```python
from build123d import *

# Parameters (mm, degrees)
SKETCH1_W           = 22.5
SKETCH1_H           = 17.75
SKETCH1_W_2         = 52
SKETCH1_H_2         = 71.85
BOSS_EXTRUDE1_DEPTH = 2
BOSS_EXTRUDE2_DEPTH = 3
SKETCH1_4_W         = 80.4
SKETCH1_4_H         = 94.4
SKETCH1_4_W_2       = 76
SKETCH1_4_H_2       = 90
BOSS_EXTRUDE3_DEPTH = 26
BOSS_EXTRUDE4_DEPTH = 78.2
CUT_EXTRUDE1_START  = -78.2
SKETCH2_3_W         = 10.3
SKETCH2_3_H         = 9
CUT_EXTRUDE1_DEPTH  = 26
CUT_EXTRUDE2_DEPTH  = 26
FILLET1_R           = 1.5
SKETCH4_R           = 3
CUT_EXTRUDE3_DEPTH  = 26
SKETCH5_R           = 1.6
BOSS_EXTRUDE5_DEPTH = 6
FILLET2_R           = 1.5


with BuildPart() as part:
    # Sketch1 → Boss-Extrude1 (new body)
    with BuildSketch(Plane(origin=(0, 0, 0), x_dir=(1, 0, 0), z_dir=(0, 1, 0))):
        Polygon((-38, -26.85), (-14, -26.85), (-14, 45), (-15.5, 45), (-15.5, 27.25), (-38, 27.25), align=None)
        with Locations((-26.75, 36.125)):
            Rectangle(SKETCH1_W, SKETCH1_H)
        with Locations((12, 9.075)):
            Rectangle(SKETCH1_W_2, SKETCH1_H_2)
        Polygon((38, -45), (38, -26.85), (-14, -26.85), (-38, -26.85), (-38, -45), align=None)
    extrude(amount=BOSS_EXTRUDE1_DEPTH)

    # Sketch1<3> → Boss-Extrude2 (add)
    with BuildSketch(Plane(origin=(0, 0, 0), x_dir=(1, 0, 0), z_dir=(0, 1, 0))):
        Polygon((-38, -26.85), (-14, -26.85), (-14, 45), (-15.5, 45), (-15.5, 27.25), (-38, 27.25), align=None)
    extrude(amount=BOSS_EXTRUDE2_DEPTH)

    # Sketch1<4> → Boss-Extrude3 (add)
    with BuildSketch(Plane(origin=(0, 0, 0), x_dir=(1, 0, 0), z_dir=(0, 1, 0))):
        Rectangle(SKETCH1_4_W, SKETCH1_4_H)
        Rectangle(SKETCH1_4_W_2, SKETCH1_4_H_2, mode=Mode.SUBTRACT)
    extrude(amount=BOSS_EXTRUDE3_DEPTH)

    # Sketch2 → Boss-Extrude4 (add)
    with BuildSketch(Plane.ZY.offset(40.2)):
        with BuildLine():
            Line((28.764343606, 5.5), (26.964343606, 5.5))
            Line((26.964343606, 5.5), (26.964343606, 0))
            Line((26.964343606, 0), (41.904953918, 0))
            Line((41.904953918, 0), (47.2, 0))
            Line((47.2, 0), (47.2, 5.5375))
            Line((47.2, 5.5375), (45, 5.5375))
            Line((45, 5.5375), (43.114695317, 5.5375))
            ThreePointArc((43.114695317, 5.5375), (35.948714495, 2.000030985), (28.764343606, 5.5))
        make_face()
    extrude(amount=-BOSS_EXTRUDE4_DEPTH)

    # Sketch2<3> → Cut-Extrude1 (cut)
    with BuildSketch(Plane.ZY.offset(40.2).offset(CUT_EXTRUDE1_START)):
        with Locations((10.914343606, 17.8)):
            Rectangle(SKETCH2_3_W, SKETCH2_3_H)
    extrude(amount=-CUT_EXTRUDE1_DEPTH, mode=Mode.SUBTRACT)

    # Sketch3 → Cut-Extrude2 (cut)
    with BuildSketch(Plane.ZY.offset(40.2)):
        with BuildLine():
            Line((-39.125, 8.5), (-33.125, 8.5))
            ThreePointArc((-33.125, 8.5), (-30.375, 5.75), (-33.125, 3))
            Line((-33.125, 3), (-39.125, 3))
            ThreePointArc((-39.125, 3), (-41.875, 5.75), (-39.125, 8.5))
        make_face()
    extrude(amount=-CUT_EXTRUDE2_DEPTH, mode=Mode.SUBTRACT)

    # Fillet1
    fillet1_edges = [part.edges().sort_by_distance(p)[0] for p in [
        (39.1, 22.3, 16.064343606),
        (39.1, 13.3, 16.064343606),
        (39.1, 13.3, 5.764343606),
        (39.1, 22.3, 5.764343606),
        (0, 0, 47.2),
        (-40.2, 13, 47.2),
        (40.2, 0, 0),
        (40.2, 13, 47.2),
        (40.2, 13, -47.2),
        (-40.2, 13, -47.2),
        (-40.2, 0, 0),
        (0, 0, -47.2),
    ]]
    fillet(fillet1_edges, radius=FILLET1_R)

    # Sketch4 → Cut-Extrude3 (cut)
    with BuildSketch(Plane(origin=(0, 0, -47.2), x_dir=(-1, 0, 0), z_dir=(0, 0, -1))):
        with Locations((-3, 14.26242493)):
            Circle(SKETCH4_R)
    extrude(amount=-CUT_EXTRUDE3_DEPTH, mode=Mode.SUBTRACT)

    # Sketch5 → Boss-Extrude5 (add)
    # profile 1 of 4: a face of its own
    with BuildSketch(Plane(origin=(0, 26, 0), x_dir=(1, 0, 0), z_dir=(0, 1, 0))):
        with BuildLine():
            Line((-33.7, 45), (-33.7, 41.8))
            ThreePointArc((-33.7, 41.8), (-34.022182541, 41.022182541), (-34.8, 40.7))
            Line((-34.8, 40.7), (-38, 40.7))
            Line((-38, 40.7), (-39.1, 40.7))
            Line((-39.1, 40.7), (-39.1, 46.1))
            Line((-39.1, 46.1), (-33.7, 46.1))
            Line((-33.7, 46.1), (-33.7, 45))
        make_face()
        with Locations(Location((-36.4, 43.4, 0), (0, 0, 270))):
            Circle(SKETCH5_R, mode=Mode.SUBTRACT)
    # profile 2 of 4: a face of its own
    with BuildSketch(Plane(origin=(0, 26, 0), x_dir=(1, 0, 0), z_dir=(0, 1, 0))):
        with BuildLine():
            Line((33.7, 46.1), (33.7, 45))
            Line((33.7, 45), (33.7, 41.8))
            ThreePointArc((33.7, 41.8), (34.022182541, 41.022182541), (34.8, 40.7))
            Line((34.8, 40.7), (38, 40.7))
            Line((38, 40.7), (39.1, 40.7))
            Line((39.1, 40.7), (39.1, 46.1))
            Line((39.1, 46.1), (33.7, 46.1))
        make_face()
        with Locations(Location((36.4, 43.4, 0), (0, 0, 90))):
            Circle(SKETCH5_R, mode=Mode.SUBTRACT)
    # profile 3 of 4: a face of its own
    with BuildSketch(Plane(origin=(0, 26, 0), x_dir=(1, 0, 0), z_dir=(0, 1, 0))):
        with BuildLine():
            Line((33.7, -45), (33.7, -41.8))
            ThreePointArc((33.7, -41.8), (34.022182541, -41.022182541), (34.8, -40.7))
            Line((34.8, -40.7), (38, -40.7))
            Line((38, -40.7), (39.1, -40.7))
            Line((39.1, -40.7), (39.1, -46.1))
            Line((39.1, -46.1), (33.7, -46.1))
            Line((33.7, -46.1), (33.7, -45))
        make_face()
        with Locations(Location((36.4, -43.4, 0), (0, 0, 270))):
            Circle(SKETCH5_R, mode=Mode.SUBTRACT)
    # profile 4 of 4: a face of its own
    with BuildSketch(Plane(origin=(0, 26, 0), x_dir=(1, 0, 0), z_dir=(0, 1, 0))):
        with BuildLine():
            Line((-33.7, -46.1), (-33.7, -45))
            Line((-33.7, -45), (-33.7, -41.8))
            ThreePointArc((-33.7, -41.8), (-34.022182541, -41.022182541), (-34.8, -40.7))
            Line((-34.8, -40.7), (-38, -40.7))
            Line((-38, -40.7), (-39.1, -40.7))
            Line((-39.1, -40.7), (-39.1, -46.1))
            Line((-39.1, -46.1), (-33.7, -46.1))
        make_face()
        with Locations(Location((-36.4, -43.4, 0), (0, 0, 270))):
            Circle(SKETCH5_R, mode=Mode.SUBTRACT)
    extrude(amount=-BOSS_EXTRUDE5_DEPTH)

    # Fillet2
    fillet2_edges = [part.edges().sort_by_distance(p)[0] for p in [
        (-33.7, 23, -45),
        (-38, 23, -40.7),
        (33.7, 23, -45),
        (38, 23, -40.7),
        (38, 23, 40.7),
        (33.7, 23, 45),
        (-33.7, 23, 45),
        (-38, 23, 40.7),
    ]]
    fillet(fillet2_edges, radius=FILLET2_R)


solid = part.part
```
CAD build for the part. Positions are in the model's coordinates, mm. A direction names the side the tool comes from. Round coordinates to 2 decimals unless told otherwise and drop trailing zeros. Order: outer loops, then holes, each group sorted by start corner. A loop starts at its lowest first (then second) coordinate and runs counter-clockwise, first axis right, second up. Notation, with made-up numbers: (77, -34.75) - (99, -34.75) arc R16 cw to (99, -28.75) - close; hole circle Ø10 at (17, 17.5). An arc over 180 degrees is marked (long way). Answer in a Markdown table with one row per item. Add a question column.
(1) Mould opens along Z. For faces 4 (the face through (-1, 0, -1)), 5 (the face through (-1, 14, -47.2)), 6 (the face through (-39.115, 5.69, -41.874)) say: +Z half, -Z half, draft (parallel to the pull), parting line (faces both ways), or undercut.
(2) Band-saw the part on A-A on z = 9. List the corners of the cut face in (x, y).
(3) Probe L1, parallel to Z at x = 36.4, y = 22; L2, parallel to X at y = 23.85, z = 43.4; L3, parallel to Z at x = -8, y = 15.25. List the from-to ranges inside material, lowest first. Write a range as [from, to].
(4) Band-saw the part on D-D on z = 32.5. List the corners of the cut face in (x, y), and give its area (3 significant figures).
(5) Band-saw the part on C-C on y = 16. List the corners of the cut face in (x, z).
(6) 3-axis set-ups, long thin cutter, end or side, ignore diameter. For faces 1 (the face through (-39.115, 5.81, -30.376)), 2 (the face through (-34.814, 23.042, 43.192)), 3 (the face through (39, 22.3, 11)): which of +Z, -Z, +X, -X, +Y, -Y reach the whole face in a straight line?
(7) Drop flat-ended pins along their axis: pin 1 Ø3.5 at (x, z) = (-36.4, -43.4) entering from +Y; pin 2 Ø1.5 at (x, z) = (7.5, 34.5) entering from +Y; pin 3 Ø9 at (x, z) = (-23.5, -38.5) entering from +Y; pin 4 Ø8 at (x, z) = (8.5, 23) entering from +Y. Give the stop position or say it passes through.
Data:
| question | item | result |
|---|---|---|
| 1 | face 4 | draft |
| 1 | face 5 | -Z half |
| 1 | face 6 | undercut |
| 2 | outline | (-40.2, 1.5) arc R1.5 ccw to (-38.7, 0) - (38.7, 0) arc R1.5 ccw to (40.2, 1.5) - (40.2, 13.3) - (38, 13.3) - (38, 2) - (-14, 2) - (-14, 3) - (-38, 3) - (-38, 26) - (-40.2, 26) - close; (38, 22.3) - (40.2, 22.3) - (40.2, 26) - (38, 26) - close |
| 3 | L1 | z = [-47.2, -45], [-41.8, -40.7], [40.7, 41.8], [45, 47.2] |
| 3 | L2 | x = [-40.2, -38], [-34.8, -33.7], [33.7, 34.8], [38, 40.2] |
| 3 | L3 | z = [-47.2, -45], [45, 47.2] |
| 4 | outline | (-40.2, 1.5) arc R1.5 ccw to (-38.7, 0) - (38.7, 0) arc R1.5 ccw to (40.2, 1.5) - (40.2, 26) - (38, 26) - (38, 2.67) - (-38, 2.67) - (-38, 26) - (-40.2, 26) - close |
| 4 | area | 316 mm^2 |
| 5 | outline | (-40.2, -45.7) arc R1.5 ccw to (-38.7, -47.2) - (0.55, -47.2) - (0.55, -45) - (-38, -45) - (-38, 45) - (38, 45) - (38, 16.06) - (40.2, 16.06) - (40.2, 45.7) arc R1.5 ccw to (38.7, 47.2) - (-38.7, 47.2) arc R1.5 ccw to (-40.2, 45.7) - close; (5.45, -47.2) - (38.7, -47.2) arc R1.5 ccw to (40.2, -45.7) - (40.2, 5.76) - (38, 5.76) - (38, -45) - (5.45, -45) - close |
| 6 | face 1 | -X |
| 6 | face 2 | +Y |
| 6 | face 3 | +X |
| 7 | pin 1 | stops at y = 26 |
| 7 | pin 2 | stops at y = 2.26 |
| 7 | pin 3 | stops at y = 2 |
| 7 | pin 4 | stops at y = 5.5 |
